Model file for the job. Use its own axes, mm. Give positions to 0.01 mm unless a question says otherwise; leave off trailing zeros. Order: outer loops, then holes, each group sorted by start corner. A loop starts at its lowest first (then second) coordinate and runs counter-clockwise, first axis right, second up. Notation, with made-up numbers: (22.5, 78.25) - (33.5, 78.25) arc R29 cw to (33.5, 112.25) - close; hole circle Ø2 at (21.5, -38.75). An arc over 180 degrees is marked (long way). Use CSV: the item, a comma, the result in double quotes. Start each with the question number.
(1) Probe L1, parallel to Y at x = 5.25, z = 521.5; L2, parallel to Z at x = 16, y = 1123.5; L3, parallel to Y at x = 3, z = 749. List the from-to ranges inside material, lowest first.
(2) Band-saw the part on A-A, the plane x = 4.25. Give the cut face in (y, z).
(3) Band-saw the part on C-C, the plane z = 875.5. Give the cut face in (x, y).
(4) Drop a flat-ended pin along its axis: pin 1 Ø3 at (x, z) = (4.5, 555.5) entering from +Y. Give the stop position or say it passes through.
(5) Band-saw the part on B-B, the plane y = 1258. Give the cut face in (x, z), then the cut area to 3 significant figures.
from build123d import *

# Parameters (mm, degrees)
F1_DEPTH = 19.05


with BuildPart() as f1:
    # F0 (on Right) → F1 (new body)
    with BuildSketch(Plane.YZ):
        with BuildLine():
            Line((0, 660.4), (0, 0))
            Line((0, 0), (2032, 0))
            Line((2032, 0), (2032, 503.370324))
            ThreePointArc((2032, 503.370324), (1890.268319, 894.153379), (1530.978359, 1103.222722))
            Line((1530.978359, 1103.222722), (609.6, 1270))
            ThreePointArc((609.6, 1270), (178.547706, 1091.452294), (0, 660.4))
        make_face()
    extrude(amount=F1_DEPTH)


solid = f1.part
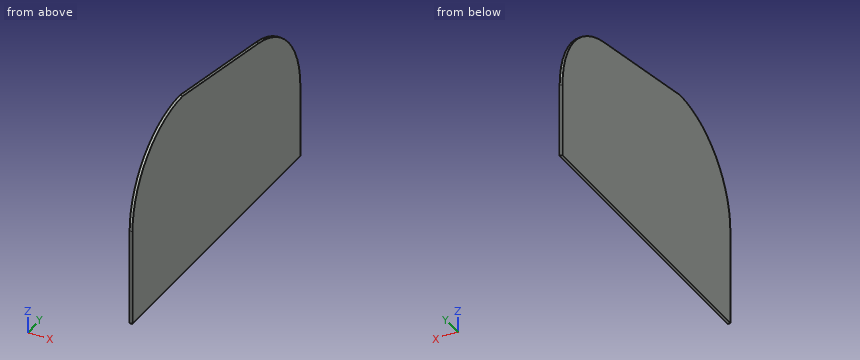
Answer block:
1,L1,"y = 0 to 2031.73"
1,L2,"z = 0 to 1176.98"
1,L3,"y = 6.47 to 1980.32"
2,outline,"(0, 0) - (2032, 0) - (2032, 503.37) arc R609.6 ccw to (1530.98, 1103.22) - (609.6, 1270) arc R609.6 ccw to (0, 660.4) - close"
3,outline,"(0, 39.21) - (19.05, 39.21) - (19.05, 1905.24) - (0, 1905.24) - close"
4,pin 1,"stops at y = 2029.89"
5,outline,"(0, 0) - (19.05, 0) - (19.05, 1152.63) - (0, 1152.63) - close"
5,area,"22,000 mm2"
